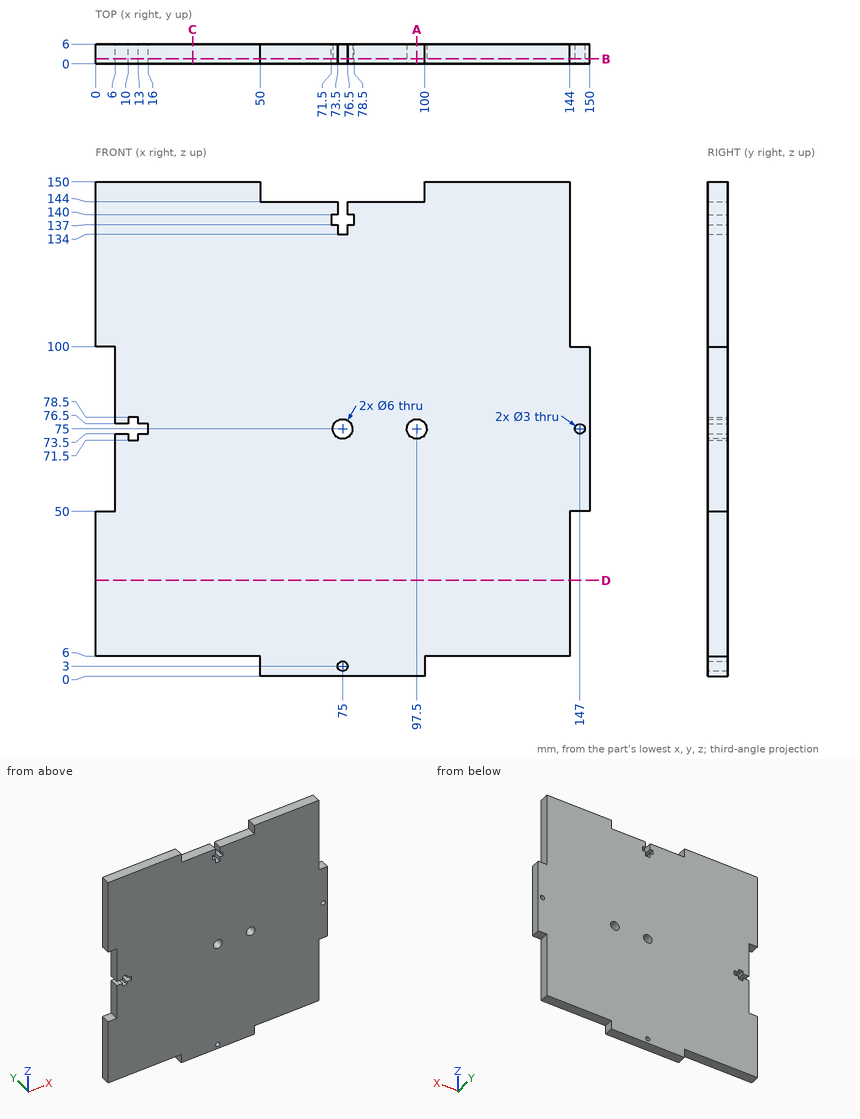
Check sheet for the drawn part. Datum: minimum x, y, z corner. Units: mm. Round coordinates to 2 decimals unless told otherwise and drop trailing zeros. Order: outer loops, then holes, each group sorted by start corner. A loop starts at its lowest first (then second) coordinate and runs counter-clockwise, first axis right, second up.
(1) Cross-section at C-C, the plane x = 29.5. Enter the section's corners in (y, z), and give its area (3 significant figures).
(2) Cross-section at B-B, the plane y = 1.5. State how many separate pieces and enclosed holes the cut face has, and give its area (3 significant figures).
(3) Cross-section at D-D, the plane z = 29. Enter the section's corners in (x, y).
(4) Go/stop test with flat-tipped pins: P1, Ø3.5, axis at y = 3, z = 135, coming from the -X side; P2, Ø1, axis at x = 33, y = 3.5, coming from the -Z side; P3, Ø2, axis at y = 3, z = 72.5, coming from the -X side; P4, Ø1.8, axis at x = 147.5, y = 3, coming from the +Z side. Record where each tip stops, or that it passes through.
(5) Cross-section at A-A, the plane x = 97.5. Enter the section's corners in (y, z).
(6) Scan lines: probe 1 along X at (y, z) = (2.3, 75); probe 2 along Z at (x, y) = (18, 2.8); probe 3 along X at (y, z) = (5.35, 22). Record each from-to range of solid material in increasing order.
Check sheet entries:
1. outline: (0, 6) - (6, 6) - (6, 150) - (0, 150) - close
1. area: 864 mm2
2. separate pieces: 1
2. enclosed holes: 4
2. area: 20,600 mm2
3. outline: (0, 0) - (144, 0) - (144, 6) - (0, 6) - close
4. P1: stops at x = 0
4. P2: stops at z = 6
4. P3: stops at x = 6
4. P4: stops at z = 100
5. outline: (0, 0) - (6, 0) - (6, 72) - (0, 72) - close; (0, 78) - (6, 78) - (6, 144) - (0, 144) - close
6. probe 1: x = 16 to 72, 78 to 94.5, 100.5 to 145.5, 148.5 to 150
6. probe 2: z = 6 to 150
6. probe 3: x = 0 to 144
